```python
from build123d import *

# Parameters (mm, degrees)
PAD026_DEPTH            = 4
SKETCH054_R             = 3.25
POCKET017_DEPTH         = 3.5
SKETCH056_R             = 1.25
POCKET018_DEPTH         = 5
FILLET001_R             = 3
BODY040_PLACEMENT_ANGLE = 90


with BuildPart() as part:
    # Sketch052 → Pad026 (new body, symmetric)
    with BuildSketch(Plane.YZ.offset(-96)):
        Polygon((93, 26.9), (93.000001, 25.221294), (97.999998, 23.199999), (101.000002, 23.2), (101, 26.9), align=None)
    extrude(amount=PAD026_DEPTH, both=True)

    # Sketch054 (on Face5 of Pad026) → Pocket017 (cut)
    with BuildSketch(Plane(origin=(0, 0, 21.9), x_dir=(0, -1, 0), z_dir=(0, 0, 1))):
        with Locations((-97, -96)):
            Circle(SKETCH054_R)
    extrude(amount=POCKET017_DEPTH, mode=Mode.SUBTRACT)

    # Sketch056 → Pocket018 (cut)
    with BuildSketch(Plane.XY.offset(22)):
        with Locations((-96, 97)):
            Circle(SKETCH056_R)
    extrude(amount=POCKET018_DEPTH, mode=Mode.SUBTRACT)

    # Fillet001
    fillet001_edges = [part.edges().sort_by_distance(p)[0] for p in [
        (-92, 93.000001, 26.060647),
        (-100, 93.000001, 26.060647),
    ]]
    fillet(fillet001_edges, radius=FILLET001_R)


with BuildPart() as part_1:
    # Body040 placement: moved
    add(part.part.moved(Location((-122, 0, 111))).rotate(Axis((-122, 0, 111), (0, -1, 0)), BODY040_PLACEMENT_ANGLE))


with BuildPart() as part_2:
    # Body046 placement: moved
    add(part_1.part.moved(Location((192, 0, 0))))


solid = part_2.part
```
Geometry check sheet. Reference: the model listing, model coordinates, mm. A direction names the side the tool comes from. Coordinates: 2 decimals unless noted, no trailing zeros. Order: outer loops, then holes, each group sorted by start corner. A loop starts at its lowest first (then second) coordinate and runs counter-clockwise, first axis right, second up. Notation, with made-up numbers: (55, -15) - (79, -15) arc R12 cw to (79, -1) - close; hole circle Ø1 at (42.25, 43). An arc over 180 degrees is marked (long way). Answer in a Markdown table with one row per item. Add a question column.
1. Draft check along Z on faces 1 (the face through (44.96, 93.45, 15.31)), 2 (the face through (44.245, 94.252, 11.562)), 3 (the face through (45.471, 100.247, 15.143)). Enter one of: +Z half, -Z half, draft (parallel to the pull), parting line (faces both ways), or undercut.
2. Access from +Z, -Z, +X, -X, +Y, -Y to the whole of each face (thin tool, end or side, straight path). Record for faces 4 (the face through (44, 93, 15)), 5 (the face through (44.6, 97, 13.6)).
3. Section check D-D (y = 99.5). Enter the section's corners in (x, z).
4. Gauge pin test, flat ends, axial feed: pin 1 Ø1.5 at (x, z) = (44, 17) entering from -Y; pin 2 Ø2 at (y, z) = (94.5, 14) entering from +X; pin 3 Ø1.5 at (y, z) = (97, 15) entering from +X; pin 4 Ø3 at (y, z) = (96, 16) entering from +X. Record the tip position at first contact, or that the pin passes through.
5. Section check C-C (z = 13.25). Enter the section's corners in (x, y).
6. Section check A-A (z = 15). Enter the section's corners in (x, y), plus the area to 3 significant figures.
7. Section check B-B (y = 97). Enter the section's corners in (x, z), plus the area to 3 significant figures.
8. Material ranges on L1, parallel to Z at x = 45.05, y = 97; L2, parallel to Z at x = 44.1, y = 97; L3, parallel to Y at x = 45.3, z = 15, recorded low to high. Write a range as [from, to].
Data:
| question | item | result |
|---|---|---|
| 1 | face 1 | draft |
| 1 | face 2 | -Z half |
| 1 | face 3 | undercut |
| 2 | face 4 | +Z, -Z, +X, -X, -Y |
| 2 | face 5 | +X |
| 3 | outline | (43.1, 11) - (46.8, 11) - (46.8, 12.92) - (44.6, 12.92) - (44.6, 17.08) - (46.8, 17.08) - (46.8, 19) - (43.1, 19) - close |
| 4 | pin 1 | stops at y = 93.01 |
| 4 | pin 2 | stops at x = 45.36 |
| 4 | pin 3 | passes through |
| 4 | pin 4 | stops at x = 44.6 |
| 5 | outline | (43.1, 93.1) - (44.82, 93.1) - (45.29, 94.26) - (44.6, 94.26) - (44.6, 99.74) - (46.8, 99.74) - (46.8, 101) - (43.1, 101) - close |
| 6 | outline | (43.1, 93) - (44.78, 93) - (45.08, 93.75) - (44.6, 93.75) - (44.6, 95.75) - (43.1, 95.75) - close; (43.1, 98.25) - (44.6, 98.25) - (44.6, 100.25) - (46.8, 100.25) - (46.8, 101) - (43.1, 101) - close |
| 6 | area | 10.1 mm² |
| 7 | outline | (43.1, 11) - (46.4, 11) - (46.4, 11.75) - (44.6, 11.75) - (44.6, 13.75) - (43.1, 13.75) - close; (43.1, 16.25) - (44.6, 16.25) - (44.6, 18.25) - (46.4, 18.25) - (46.4, 19) - (43.1, 19) - close |
| 7 | area | 10.9 mm² |
| 8 | L1 | z = [11, 11.75], [18.25, 19] |
| 8 | L2 | z = [11, 13.75], [16.25, 19] |
| 8 | L3 | y = [100.25, 101] |
